Source: CAD feature listing. Evaluate the final solid. Frame: model axes, mm. A direction names the side the tool comes from. Give positions to 0.01 mm unless a question says otherwise; leave off trailing zeros. Order: outer loops, then holes, each group sorted by start corner. A loop starts at its lowest first (then second) coordinate and runs counter-clockwise, first axis right, second up. Notation, with made-up numbers: M 25,45 L 79,45 A16 ccw 79,74 Z; hole C 45.25,-20.5 d8. An arc over 180 degrees is marked long. Use CSV: the item, a comma, the result in double quotes. Start each with the question number.
1. Section query C-C, the plane y = 3. Return the cut outline in (x, z), plus the area to 3 significant figures.
2. Reachability of faces 4 (the flat face through (-9, 0, -36)), 5 (the flat face through (-3, 4, -12)), 6 (the flat face through (-15, 4, -53)) from +Z, -Z, +X, -X, +Y, -Y: full face, straight path, thin tool, end or side. Return the list, or none.
3. Pin query (flat end, axial travel): P1, Ø4, axis at y = 4, z = -52.5, coming from the +X side; P2, Ø4, axis at y = 3, z = -14.5, coming from the -X side; P3, Ø3, axis at x = -7, y = 3, coming from the +Z side; P4, Ø4, axis at x = -4, z = -17.5, coming from the -Y side. Return the tip coordinate at first contact, or that it passes through.
4. Section query B-B, the plane x = -17.25. Return the cut outline in (y, z), plus the area to 3 significant figures.
5. Line query: line 1 along Y through (x, z) = (-1.35, -4); line 2 along Y through (x, z) = (-18.05, -57.5); line 3 along X through (y, z) = (5, -54). Output: solid intervals per line, ascending. Write a range as [from, to].
6. Section query A-A, the plane z = -57.5. Return the cut outline in (x, y).
7. Mould query, pull axis Y, two halves, no side actions, for faces 1 (the flat face through (-11, 4, -33)), 2 (the flat face through (-9, 8, -36)), 3 (the cylindrical face through (-1.521, 2.544, -3.405)). Classes: released by +Y, released by -Y, zero draft, split by the parting line, or undercut.
8. Section query D-D, the plane z = -4. Return the cut outline in (x, y), plus the area to 3 significant figures.
from build123d import *

# Parameters (mm, degrees)
BOSS_EXTRUDE1_DEPTH     = 8
SKETCH2_R               = 2.25
SKETCH2_R_2             = 0.75
CUT_EXTRUDE1_DEPTH      = 16
CUT_EXTRUDE1_DEPTH_BACK = 5


with BuildPart() as part:
    # Sketch1 → Boss-Extrude1 (new body)
    with BuildSketch(Plane(origin=(0, 0, 0), x_dir=(1, 0, 0), z_dir=(0, 1, 0))):
        Polygon((0, 0), (-3, 0), (-3, 25), (-19, 41), (-19, 62.5), (-15, 62.5), (-15, 44.071067812), (0, 29.071067812), align=None)
    extrude(amount=BOSS_EXTRUDE1_DEPTH)

    # Sketch2 → Cut-Extrude1 (cut, two sides)
    with BuildSketch(Plane(origin=(-15, 0, 0), x_dir=(0, 0, -1), z_dir=(1, 0, 0))) as cut_extrude1_sk:
        with Locations((57.5, 4)):
            Circle(SKETCH2_R)
        with Locations((4, 3)):
            Circle(SKETCH2_R_2)
    extrude(amount=CUT_EXTRUDE1_DEPTH, mode=Mode.SUBTRACT)
    extrude(cut_extrude1_sk.sketch, amount=-CUT_EXTRUDE1_DEPTH_BACK, mode=Mode.SUBTRACT)


solid = part.part
Result set:
1,outline,"M -19,-62.5 L -15,-62.5 L -15,-59.52 L -19,-59.52 Z; M -19,-55.48 L -15,-55.48 L -15,-44.07 L 0,-29.07 L 0,-4.75 L -3,-4.75 L -3,-25 L -19,-41 Z; M -3,-3.25 L 0,-3.25 L 0,0 L -3,0 Z"
1,area,"250 mm2"
2,face 4,"+Z, -Z, +X, -X, -Y"
2,face 5,"+Z, -X, +Y, -Y"
2,face 6,"-Z, +X, +Y, -Y"
3,P1,"x = -15"
3,P2,"x = -3"
3,P3,"z = -27.5"
3,P4,"y = 0"
4,outline,"M 0,-62.5 L 8,-62.5 L 8,-39.25 L 0,-39.25 Z; hole C 4,-57.5 d4.5"
4,area,"170 mm2"
5,line 1,"[0, 2.25], [3.75, 8]"
5,line 2,"[0, 1.75], [6.25, 8]"
5,line 3,"[-19, -15]"
6,outline,"M -19,0 L -15,0 L -15,1.75 L -19,1.75 Z; M -19,6.25 L -15,6.25 L -15,8 L -19,8 Z"
7,face 1,"zero draft"
7,face 2,"released by +Y"
7,face 3,"undercut"
8,outline,"M -3,0 L 0,0 L 0,2.25 L -3,2.25 Z; M -3,3.75 L 0,3.75 L 0,8 L -3,8 Z"
8,area,"19.5 mm2"
